Autodesk Inventor part; units mm, degrees
ref_plane "作業平面1" through (8.6603, 7.5, -88) normal (0, 0, 1) x (1, 0, 0)
ref_plane "作業平面2" through (13.4603, 7.5, -88) normal (-1, 0, 0) x (0, 0, 1)
ref_plane "作業平面3" through (0, 0, 0) normal (0, 0, 1) x (1, 0, 0)
sketch "スケッチ1" plane through (0, 0, 0) normal (0, 1, 0) x (-1, 0, 0)
  arc A0 (0, 57) -> (0, -57) centre (0, 0) ccw
  line L0 (0, 57) -> (0, 93) construction
  line L1 (0, 57) -> (0, 93)
  line L2 (0, 93) -> (-80.5404, 46.5)
  line L3 (-80.5404, 46.5) -> (-100.5404, 46.5)
  line L4 (-100.5404, 46.5) -> (-100.5404, 110)
  line L5 (-100.5404, 110) -> (-110.5404, 110)
  line L6 (-110.5404, 110) -> (-110.5404, 0)
  line L7 (0, -57) -> (0, -93) construction
  line L8 (0, -93) -> (-80.5404, -46.5)
  line L9 (-80.5404, -46.5) -> (-100.5404, -46.5)
  line L10 (-100.5404, -46.5) -> (-100.5404, -110)
  line L11 (-100.5404, -110) -> (-110.5404, -110)
  line L12 (-110.5404, -110) -> (-110.5404, 0)
  line L13 (0, -93) -> (0, -57)
  dimension "d0" = 57
  dimension "d7" = 10
sketch "スケッチ2" plane through (0, 0, 0) normal (0, 1, 0) x (-1, 0, 0)
  point P0 (0, 0)
extrude "押し出し1" add sketch "スケッチ1" along normal blind 15
sketch "スケッチ3" plane through (100.5404, 0, 46.5) normal (-1, 0, 0) x (0, 0, 1)
  point P0 (-46.5, 0)
sketch "スケッチ4" plane through (0, 0, 57) normal (-1, 0, 0) x (0, 0, 1)
  line L0 (0, 0) -> (0, 15)
  line L1 (0, 0) -> (31, 0)
  line L2 (36, 0) -> (36, 15)
  line L3 (31, 0) -> (31, 7.5)
  point P0 (-57, 0)
  dimension "d10" = 31
  dimension "d11" = 7.5
hole "穴1" at (0, 7.5, 88) direction (1, 0, 0) diameter 2.459 depth 31.54 tip angle 118
sketch "スケッチ5" plane through (0, 0, -93) normal (-1, 0, 0) x (0, 0, 1)
  line L0 (36, 0) -> (36, 15)
  line L1 (36, 0) -> (5, 0)
  line L2 (-17, 0) -> (46.5, 0)
  line L3 (5, 0) -> (5, 7.5)
  line L4 (-17, 15) -> (46.5, 15)
  point P0 (93, 0)
  dimension "d19" = 31
  dimension "d20" = 7.5
hole "穴2" at (0, 7.5, -88) direction (1, 0, 0) diameter 2.459 depth 35.79 tip angle 118
sketch "スケッチ7" plane through (0, 0, -93) normal (0.5, 0, -0.866) x (-0.866, 0, -0.5)
  ellipse E0 centre (-10, 7.5) end of major axis (-12.459, 7.5) minor radius 1.2295
  point P0 (-46.5, 0)
  point P1 (-10, 7.5)
ref_plane "作業平面1" through (8.6603, 7.5, -88) normal (0, 0, 1) x (1, 0, 0)
sketch "スケッチ8" plane through (8.6603, 7.5, -88) normal (0, 0, 1) x (1, 0, 0)
  ellipse E0 centre (0, 0) end of major axis (-2.1296, 0) minor radius 1.2295
  line L0 (0, 0) -> (4.8, 0)
  point P0 (-8.6603, -7.5)
  dimension "d28" = 4.8
ref_plane "作業平面2" through (13.4603, 7.5, -88) normal (-1, 0, 0) x (0, 0, 1)
sketch "スケッチ9" plane through (13.4603, 7.5, -88) normal (-1, 0, 0) x (0, 0, 1)
  point P0 (88, -7.5)
  point P1 (0, 0)
hole "穴3" at (13.4603, 7.5, -88) direction (-1, 0, 0) diameter 2.459 end through all counterbore diameter 5.5 counterbore depth 5
sketch "スケッチ10" plane through (100.5404, 0, 46.5) normal (-1, 0, 0) x (0, 0, 1)
  line L0 (63.5, 0) -> (63.5, 15)
  line L1 (63.5, 7.5) -> (57, 7.5)
  line L2 (46.5, 0) -> (46.5, 15)
  line L3 (57, 7.5) -> (25, 7.5)
  point P0 (-46.5, 0)
  dimension "d36" = 6.5
  dimension "d37" = 32
hole "穴4" at (100.5404, 7.5, 103.5) at (100.5404, 7.5, 71.5) direction (1, 0, 0) diameter 4.134 end through all counterbore diameter 9 counterbore depth 1
ref_plane "作業平面3" through (0, 0, 0) normal (0, 0, 1) x (1, 0, 0)
mirror "ミラー1" about plane through (0, 0, 0) normal (0, 0, 1) of "穴4", "穴3"
properties part number "nowtrying"
Work out the finished part from the listing and answer in its coordinate system (mm). A direction names the side the tool comes from. Round coordinates to 2 decimals unless told otherwise and drop trailing zeros. Write each loop counter-clockwise with the first axis right and the second up, starting at its lowest first coordinate (ties: lowest second). Pieces come first, ordered by that corner, then holes. Notation, with made-up numbers: M 9.5,40.5 L 25.5,40.5 A24 ccw 25.5,50.5 Z; hole C -27.5,-23.75 d2. An arc over 180 degrees is marked long. Use a Markdown table: item, result.
1) Determine the mould class of faces 6 (the face through (106.103, 7.591, -101.435)), 7 (the face through (101.54, 8, -74)), 8 (the face through (101.54, 8, -106)) for opening direction X: pulls with the +X half, pulls with the -X half, needs draft (parallel to the pull), parting line crosses it, or undercut.
Taken from the geometry:
| item | result |
|---|---|
| face 6 | needs draft |
| face 7 | undercut |
| face 8 | pulls with the -X half |
2) The part is cut by section D-D on x = 77. Give the vertices of the cut face in (y, z), plus the area to 3 significant figures.
Taken from the geometry:
| item | result |
|---|---|
| outline | M 0,-48.54 L 15,-48.54 L 15,48.54 L 0,48.54 Z |
| area | 1,460 mm2 |
3) The part is cut by section B-B on z = 0. Give the vertices of the cut face in (x, y), plus the area to 3 significant figures.
Taken from the geometry:
| item | result |
|---|---|
| outline | M 57,0 L 110.54,0 L 110.54,15 L 57,15 Z |
| area | 803 mm2 |
4) Which of the six approach directions +Z, -Z, +X, -X, +Y, -Y give full straight-line access (tool end or side, diameter ignored) to faces 1 (the face through (39.706, 7.395, -70.075)), 2 (the face through (106.103, 7.591, -69.435)), 3 (the face through (39.706, 7.395, 70.075)), 4 (the face through (101.54, 8, 101)), 5 (the face through (101.54, 8, 69))?
Taken from the geometry:
| item | result |
|---|---|
| face 1 | -Z, +Y, -Y |
| face 2 | +X |
| face 3 | +Z, +Y, -Y |
| face 4 | -X |
| face 5 | none |
5) The part is cut by section A-A on x = 47.5. Give the vertices of the cut face in (y, z).
Taken from the geometry:
| item | result |
|---|---|
| outline | M 0,-65.58 L 15,-65.58 L 15,-31.51 L 0,-31.51 Z; M 0,31.51 L 15,31.51 L 15,65.58 L 0,65.58 Z |
6) Flat-ended cylindrical pins translate along their axes: pin 1 (1 mm diameter, centred on y = 8.5, z = 39.5, fed in from -X); pin 2 (7 mm diameter, centred on y = 6.5, z = -103, fed in from -X); pin 3 (4 mm diameter, centred on x = 35.5, y = 12.5, fed in from -Z). Find the tip coordinate at first contact, or state that the pin passes through.
Taken from the geometry:
| item | result |
|---|---|
| pin 1 | stops at x = 40.61 |
| pin 2 | stops at x = 100.54 |
| pin 3 | stops at z = -73.66 |
7) Consider line 1 (Z direction, x = 105, y = 7.5); line 2 (Z direction, x = 101.1, y = 7.5); line 3 (Y direction, x = 107, z = -71.5). Determine where each line is inside the solid, lowest interval first. Write a range as [from, to].
Taken from the geometry:
| item | result |
|---|---|
| line 1 | z = [-110, -105.57], [-101.43, -73.57], [-69.43, 69.43], [73.57, 101.43], [105.57, 110] |
| line 2 | z = [-110, -108], [-99, -76], [-67, 67], [76, 99], [108, 110] |
| line 3 | y = [0, 5.43], [9.57, 15] |
8) The part is cut by section C-C on x = 32. Give the vertices of the cut face in (y, z).
Taken from the geometry:
| item | result |
|---|---|
| outline | M 0,-74.52 L 15,-74.52 L 15,-47.17 L 0,-47.17 Z; M 0,47.17 L 15,47.17 L 15,74.52 L 0,74.52 Z |
